Build history of the part. All positions in model axes, mm. Face numbers are marked on the shaded views. Give positions to 0.01 mm unless a question says otherwise; leave off trailing zeros. Order: outer loops, then holes, each group sorted by start corner. A loop starts at its lowest first (then second) coordinate and runs counter-clockwise, first axis right, second up. Notation, with made-up numbers: (39.5, 5.25) -> (75.5, 5.25) arc R34 ccw to (75.5, 41.25) -> close; hole circle Ø2 at (87.25, 84). An arc over 180 degrees is marked (long way). Write item = value, one per line. Start each with the question number.
from build123d import *

# Parameters (mm, degrees)
SKETCH1_R           = 1.5875
BOSS_EXTRUDE1_DEPTH = 11.90625


with BuildPart() as part:
    # Sketch1 → Boss-Extrude1 (new body)
    with BuildSketch(Plane.XY):
        with BuildLine():
            Line((0, 990.6), (0, 0))
            Line((0, 0), (457.201, 0))
            Line((457.201, 0), (457.201, 13.862038208))
            ThreePointArc((457.201, 13.862038208), (232.767577124, 176.628269142), (124.367415652, 431.8))
            Line((124.367415652, 431.8), (50.8, 990.6))
            Line((50.8, 990.6), (0, 990.6))
        make_face()
        with Locations((18.25625, 18.25625)):
            Circle(SKETCH1_R, mode=Mode.SUBTRACT)
        with Locations((18.25625, 43.65625)):
            Circle(SKETCH1_R, mode=Mode.SUBTRACT)
        with Locations((56.35625, 63.5)):
            Circle(SKETCH1_R, mode=Mode.SUBTRACT)
        with Locations((56.35625, 101.6)):
            Circle(SKETCH1_R, mode=Mode.SUBTRACT)
        with Locations((388.14375, 18.25625)):
            Circle(SKETCH1_R, mode=Mode.SUBTRACT)
        with Locations((18.25625, 972.34375)):
            Circle(SKETCH1_R, mode=Mode.SUBTRACT)
    extrude(amount=BOSS_EXTRUDE1_DEPTH)


solid = part.part
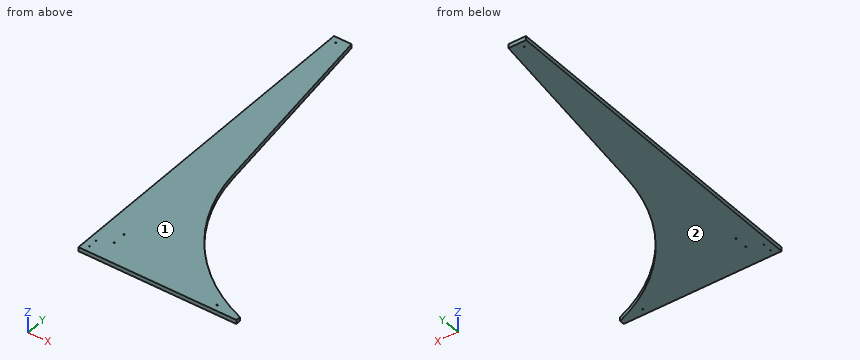
(1) Cut at B-B, the plane y = 476. Give the cut face in (x, z).
(2) Mould opens along Z. For the marked faces 1 and 2 say: released by +Z, released by -Z, zero draft, split by the parting line, or undercut.
(3) Cut at A-A, the plane z = 9.25. Give the cut face in (x, y) (1 decimal).
(4) Wall check: line 1 (X direction, y = 101.6, z = 5); line 2 (Y direction, x = 271, z = 1.75); line 3 (X direction, y = 917, z = 7.5). Give the ranges that are in metal, low to high. Write a range as [from, to].
(5) Flat gauge pins, fed straight in: P1, Ø2.5, axis at x = 56.36, y = 101.6, coming from the +Z side; P2, Ø3.5, axis at x = 18.26, y = 43.66, coming from the -Z side; P3, Ø1, axis at x = 410.5, z = 6.5, coming from the +Y side; P4, Ø1.5, axis at y = 464.5, z = 6, coming from the +X side. Where does each tip first touch, or does it go through?
(6) Cut at C-C, the plane x = 93. Give the cut face in (y, z), plus the area to 3 significant figures.
Results:
q1.outline = (0, 0) -> (118.55, 0) -> (118.55, 11.91) -> (0, 11.91) -> close
q2.face_1 = released by +Z
q2.face_2 = released by -Z
q3.outline = (0, 0) -> (457.2, 0) -> (457.2, 13.9) arc R518.2 cw to (124.4, 431.8) -> (50.8, 990.6) -> (0, 990.6) -> close; hole circle Ø3.2 at (18.3, 18.3); hole circle Ø3.2 at (18.3, 43.7); hole circle Ø3.2 at (18.3, 972.3); hole circle Ø3.2 at (56.4, 63.5); hole circle Ø3.2 at (56.4, 101.6); hole circle Ø3.2 at (388.1, 18.3)
q4.line_1 = [0, 54.77], [57.94, 306.09]
q4.line_2 = [0, 133.73]
q4.line_3 = [0, 60.49]
q5.P1 = through
q5.P2 = 0
q5.P3 = 34.17
q5.P4 = 120.16
q6.outline = (0, 0) -> (670.06, 0) -> (670.06, 11.91) -> (0, 11.91) -> close
q6.area = 7,980 mm2
